Could you check a few things on this drawing? It's one solid part, dimensions in mm from its lowest x, y, z. A direction names the side the tool comes from. Give positions to 0.01 mm unless a question says otherwise; leave off trailing zeros. Loops run counter-clockwise (first coordinate to the right, second up) from the corner with the lowest first, then second, coordinate; pieces in that order, holes last. Notation, with made-up numbers: M -1.5,-7 L 6.5,-7 A9 cw 6.5,2 Z; hole C 64,45.25 d2. An arc over 180 degrees is marked long. Answer in a Markdown table with one row per item. Add a question column.
1. If we section it at B-B on z = 25.5: List the corners of the cut face in (x, y) for me, then the cut area to 3 significant figures.
2. If we section it at C-C on y = 23.5: List the corners of the cut face in (x, z) for me.
3. If we section it at A-A on x = 72: List the corners of the cut face in (y, z) for me.
4. If we section it at D-D on z = 5: List the corners of the cut face in (x, y) for me.
5. Which directions (+Z, -Z, +X, -X, +Y, -Y) give clear straight access to the entire face, cutting with the end or side of a thin tool? Please do the marked faces 1 and 2.
6. I need wall thicknesses on line 1 along Z through (x, y) = (51, 12.5); line 2 along Y through (x, z) = (34.5, 85); line 3 along Y through (x, z) = (63.5, 44.5). Which ranges of each line are inside material? Lowest first, please. Write a range as from..to.
7. I'm going to push a flat-ended pin straight in: pin 1 Ø1 at (x, y) = (18.5, 13.5) entering from -Z. Where does the tip first touch, or does it pass through?
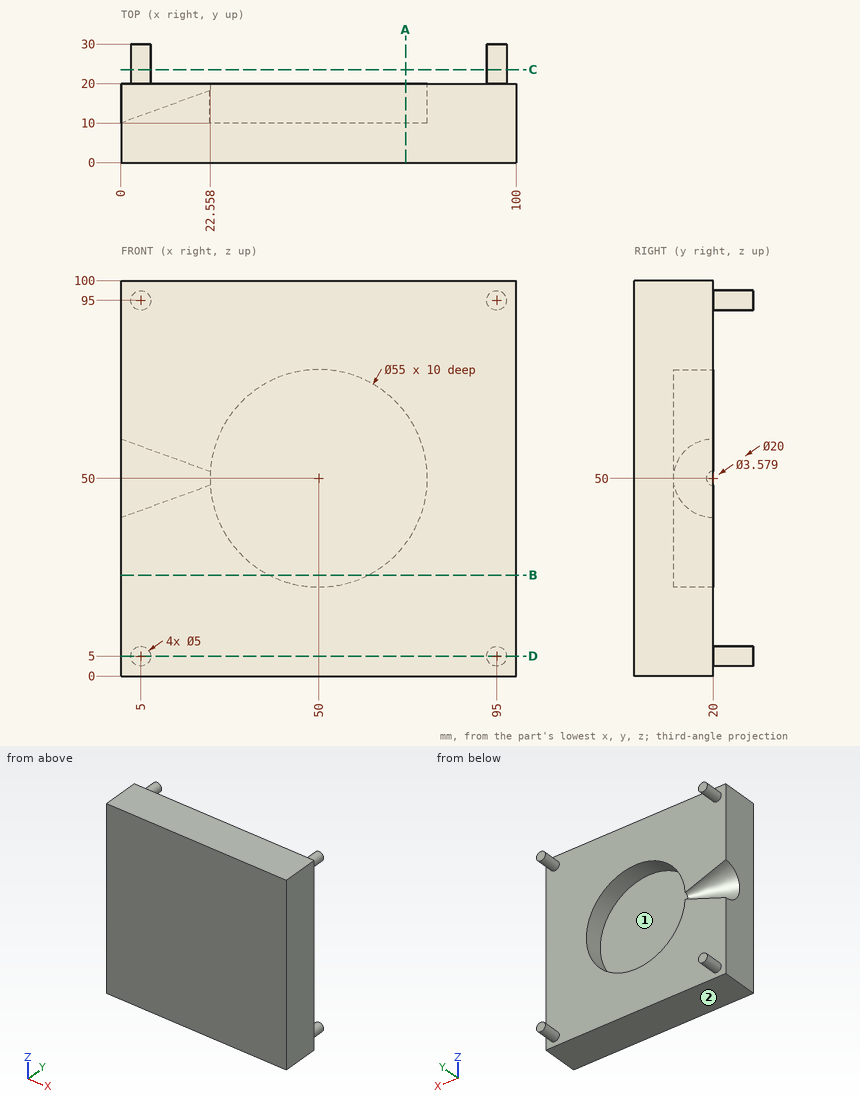
Results:
| question | item | result |
|---|---|---|
| 1 | outline | M 0,0 L 100,0 L 100,20 L 62.49,20 L 62.49,10 L 37.51,10 L 37.51,20 L 0,20 Z |
| 1 | area | 1,750 mm2 |
| 2 | outline | C 5,5 d5; C 5,95 d5; C 95,5 d5; C 95,95 d5 |
| 3 | outline | M 0,0 L 20,0 L 20,33.5 L 10,33.5 L 10,66.5 L 20,66.5 L 20,100 L 0,100 Z |
| 4 | outline | M 0,0 L 100,0 L 100,20 L 97.5,20 L 97.5,30 L 92.5,30 L 92.5,20 L 7.5,20 L 7.5,30 L 2.5,30 L 2.5,20 L 0,20 Z |
| 5 | face 1 | +Y |
| 5 | face 2 | -Z, +X, -X, +Y, -Y |
| 6 | line 1 | 0..22.52, 77.48..100 |
| 6 | line 2 | 0..20 |
| 6 | line 3 | 0..10 |
| 7 | pin 1 | z = 0 |
